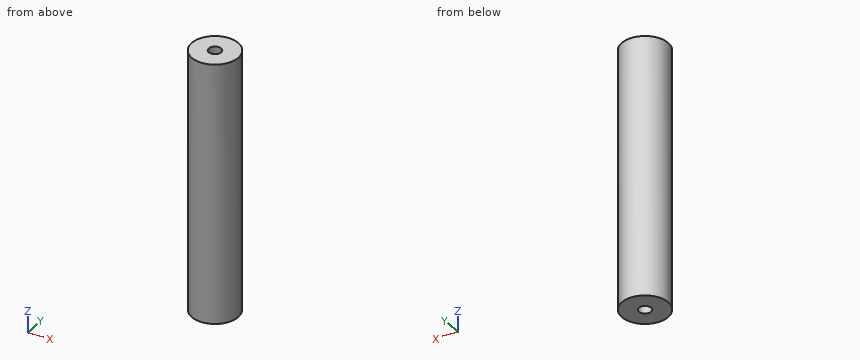
from build123d import *

# Parameters (mm, degrees)
SKETCH1_R           = 9.375
BOSS_EXTRUDE1_DEPTH = 105
SKETCH4_R           = 2.5
CUT_EXTRUDE1_DEPTH  = 20


with BuildPart() as part:
    # Sketch1 → Boss-Extrude1 (new body)
    with BuildSketch(Plane.XY):
        Circle(SKETCH1_R)
    extrude(amount=BOSS_EXTRUDE1_DEPTH)

    # Sketch4 → Cut-Extrude1 (cut)
    with BuildSketch(Plane.XY.offset(105)):
        Circle(SKETCH4_R)
    cut_extrude1 = extrude(amount=-CUT_EXTRUDE1_DEPTH, mode=Mode.SUBTRACT)

    # Mirror1: Cut-Extrude1 across plane
    add(cut_extrude1.mirror(Plane(origin=(0, 0, 52.5), x_dir=(1, 0, 0), z_dir=(0, 0, -1))), mode=Mode.SUBTRACT)


solid = part.part
Verification items for the finished model (mm, model axes). Coordinates: 2 decimals unless noted, no trailing zeros. Loops run counter-clockwise (first coordinate to the right, second up) from the corner with the lowest first, then second, coordinate; pieces in that order, holes last. Notation, with made-up numbers: M 76,-5.75 L 134,-5.75 A16 ccw 134,2.25 Z; hole C 46.25,87.5 d7. An arc over 180 degrees is marked long. One line per item, written item: value.
1. Material ranges on line 1 along Y through (x, z) = (0, 14.25) (3 decimals); line 2 along Z through (x, y) = (0.75, -1.5); line 3 along Y through (x, z) = (1, 11), recorded low to high. Write a range as from..to.
Answers follow:
line 1: -9.375..-2.5, 2.5..9.375
line 2: 20..85
line 3: -9.32..-2.29, 2.29..9.32
2. Gauge pin test, flat ends, axial feed: P1, Ø10, axis at x = 1, z = 40.5, coming from the -Y side (3 decimals); P2, Ø1.5, axis at x = 1, y = 0.5, coming from the +Z side; P3, Ø4, axis at x = -3.5, z = 73, coming from the -Y side; P4, Ø3, axis at x = 0, y = 0, coming from the -Z side. Record the tip position at first contact, or that the pin passes through.
Answers follow:
P1: y = -9.375
P2: z = 85
P3: y = -9.25
P4: z = 20
3. Section check C-C on z = 43.5. Record the cut outline in (x, y) (3 decimals), plus the area to 3 significant figures.
Answers follow:
outline: C 0,0 d18.75
area: 276 mm^2
4. Section check D-D on z = 14.5. Record the cut outline in (x, y) (3 decimals).
Answers follow:
outline: C 0,0 d18.75; hole C 0,0 d5
5. Section check A-A on x = 0. Record the cut outline in (y, z) (3 decimals), plus the area to 3 significant figures.
Answers follow:
outline: M -9.375,0 L -2.5,0 L -2.5,20 L 2.5,20 L 2.5,0 L 9.375,0 L 9.375,105 L 2.5,105 L 2.5,85 L -2.5,85 L -2.5,105 L -9.375,105 Z
area: 1,770 mm^2
